The listing builds one solid part. Answer for the finished solid, in the listing's coordinates (mm). Round coordinates to 2 decimals unless told otherwise and drop trailing zeros. Order: outer loops, then holes, each group sorted by start corner. A loop starts at its lowest first (then second) coordinate and runs counter-clockwise, first axis right, second up. Notation, with made-up numbers: (42, 64) - (76, 64) arc R32 cw to (76, 95) - close; hole circle Ø9 at (-12.5, 8.5). An arc over 180 degrees is marked (long way). One line per item, written item: value. Start each with the question number.
1. Flat-ended cylindrical pins translate along their axes: P1, Ø1.7, axis at y = 5, z = -5.5, coming from the +X side; P2, Ø6, axis at y = 6.5, z = 10, coming from the +X side; P3, Ø2.5, axis at y = 7.5, z = -5.5, coming from the -X side. Find the tip coordinate at first contact, or state that the pin passes through.
2. Straight lines are drawn through the part: line 1 (Z direction, x = 0, y = 2.5) (3 decimals); line 2 (X direction, y = 2.75, z = 0) (3 decimals); line 3 (X direction, y = 8, z = -3). For each, find the intervals that lie inside material, in ascending order.
3. For a pull along Z with two mould halves and no side action, classify faces 1 (the flat face through (0, 5, -6.731)), 2 (the flat face through (-8, 7.29, 8)) as released by +Z, released by -Z, zero draft, split by the parting line, or undercut.
4. Section B-B, the plane x = -1 is taken. Give the vertices of the cut face in (y, z).
5. Section A-A, the plane y = 0.5 is taken. Give the vertices of the cut face in (x, z) (3 decimals).
6. Section D-D, the plane x = -10 is taken. Give the vertices of the cut face in (y, z), then the cut area to 3 significant figures.
7. Section C-C, the plane z = 0.5 is taken. Give the vertices of the cut face in (x, y), then the cut area to 3 significant figures.
from build123d import *

# Parameters (mm, degrees)
SKETCH2_R           = 10.795
BOSS_EXTRUDE1_DEPTH = 10.287
SKETCH3_R           = 17.8689
BOSS_EXTRUDE2_DEPTH = 2.9972
CUT_EXTRUDE1_DEPTH  = 11.287
CUT_EXTRUDE2_DEPTH  = 11.287


with BuildPart() as part:
    # Sketch2 → Boss-Extrude1 (new body)
    with BuildSketch(Plane(origin=(0, 0, 0), x_dir=(1, 0, 0), z_dir=(0, 1, 0))):
        Circle(SKETCH2_R)
    extrude(amount=BOSS_EXTRUDE1_DEPTH)

    # Sketch3 → Boss-Extrude2 (add)
    with BuildSketch(Plane(origin=(0, 10.287, 0), x_dir=(1, 0, 0), z_dir=(0, 1, 0))):
        Circle(SKETCH3_R)
    extrude(amount=-BOSS_EXTRUDE2_DEPTH)

    # Sketch4 → Cut-Extrude1 (cut, through all)
    with BuildSketch(Plane(origin=(0, 10.287, 0), x_dir=(1, 0, 0), z_dir=(0, 1, 0))):
        with BuildLine():
            ThreePointArc((1.4e-08, 17.8689), (1.079645228, 17.410056336), (1.4986, 16.314315402))
            ThreePointArc((1.4986, 16.314315402), (3.196164746, 16.068205249), (4.858692347, 15.645951479))
            ThreePointArc((4.858692347, 15.645951479), (5.665077892, 16.497957009), (6.838131777, 16.508711064))
            ThreePointArc((6.838131777, 16.508711064), (3.486049352, 17.525554117), (1.4e-08, 17.8689))
        make_face()
        with BuildLine():
            ThreePointArc((4.858692347, 15.645951479), (3.196164746, 16.068205249), (1.4986, 16.314315402))
            ThreePointArc((1.4986, 16.314315402), (2.893978636, 14.549013087), (4.858692347, 15.645951479))
        make_face()
        with BuildLine():
            ThreePointArc((12.63522035, 12.635220375), (9.927428836, 14.857447422), (6.838131777, 16.508711064))
            ThreePointArc((6.838131777, 16.508711064), (7.660002201, 15.671632478), (7.627744082, 14.498972695))
            ThreePointArc((7.627744082, 14.498972695), (9.101907128, 13.621966658), (10.476292829, 12.595633274))
            ThreePointArc((10.476292829, 12.595633274), (11.547344433, 13.074193358), (12.63522035, 12.635220375))
        make_face()
        with BuildLine():
            ThreePointArc((10.476292829, 12.595633274), (9.101907128, 13.621966658), (7.627744082, 14.498972695))
            ThreePointArc((7.627744082, 14.498972695), (8.241353895, 12.334057732), (10.476292829, 12.595633274))
        make_face()
        with BuildLine():
            ThreePointArc((16.508710924, 6.838132115), (14.857447311, 9.927429003), (12.63522035, 12.635220375))
            ThreePointArc((12.63522035, 12.635220375), (13.074193359, 11.54734445), (12.595633274, 10.476292829))
            ThreePointArc((12.595633274, 10.476292829), (13.621966658, 9.101907128), (14.498972695, 7.627744082))
            ThreePointArc((14.498972695, 7.627744082), (15.671632308, 7.660002268), (16.508710924, 6.838132115))
        make_face()
        with BuildLine():
            ThreePointArc((14.498972695, 7.627744082), (13.621966658, 9.101907128), (12.595633274, 10.476292829))
            ThreePointArc((12.595633274, 10.476292829), (12.334057732, 8.241353895), (14.498972695, 7.627744082))
        make_face()
        with BuildLine():
            ThreePointArc((17.8689, 0), (17.525554083, 3.486049525), (16.508710924, 6.838132115))
            ThreePointArc((16.508710924, 6.838132115), (16.497957082, 5.665078059), (15.645951479, 4.858692347))
            ThreePointArc((15.645951479, 4.858692347), (16.068205249, 3.196164746), (16.314315402, 1.4986))
            ThreePointArc((16.314315402, 1.4986), (17.410056341, 1.079645223), (17.8689, 0))
        make_face()
        with BuildLine():
            ThreePointArc((16.314315402, 1.4986), (16.068205249, 3.196164746), (15.645951479, 4.858692347))
            ThreePointArc((15.645951479, 4.858692347), (14.549013087, 2.893978636), (16.314315402, 1.4986))
        make_face()
        with BuildLine():
            ThreePointArc((16.508710924, -6.838132115), (17.525554083, -3.486049525), (17.8689, 0))
            ThreePointArc((17.8689, 0), (17.410056341, -1.079645223), (16.314315402, -1.4986))
            ThreePointArc((16.314315402, -1.4986), (16.068205249, -3.196164746), (15.645951479, -4.858692347))
            ThreePointArc((15.645951479, -4.858692347), (16.497957082, -5.665078059), (16.508710924, -6.838132115))
        make_face()
        with BuildLine():
            ThreePointArc((15.645951479, -4.858692347), (16.068205249, -3.196164746), (16.314315402, -1.4986))
            ThreePointArc((16.314315402, -1.4986), (14.549013087, -2.893978636), (15.645951479, -4.858692347))
        make_face()
        with BuildLine():
            ThreePointArc((12.635220358, -12.635220367), (14.857447314, -9.927428998), (16.508710924, -6.838132115))
            ThreePointArc((16.508710924, -6.838132115), (15.671632308, -7.660002268), (14.498972695, -7.627744082))
            ThreePointArc((14.498972695, -7.627744082), (13.621966658, -9.101907128), (12.595633274, -10.476292829))
            ThreePointArc((12.595633274, -10.476292829), (13.074193359, -11.547344445), (12.635220358, -12.635220367))
        make_face()
        with BuildLine():
            ThreePointArc((12.595633274, -10.476292829), (13.621966658, -9.101907128), (14.498972695, -7.627744082))
            ThreePointArc((14.498972695, -7.627744082), (12.334057732, -8.241353895), (12.595633274, -10.476292829))
        make_face()
        with BuildLine():
            ThreePointArc((6.838132083, -16.508710938), (9.927428978, -14.857447327), (12.635220358, -12.635220367))
            ThreePointArc((12.635220358, -12.635220367), (11.547344438, -13.074193358), (10.476292829, -12.595633274))
            ThreePointArc((10.476292829, -12.595633274), (9.101907128, -13.621966658), (7.627744082, -14.498972695))
            ThreePointArc((7.627744082, -14.498972695), (7.660002262, -15.671632324), (6.838132083, -16.508710938))
        make_face()
        with BuildLine():
            ThreePointArc((7.627744082, -14.498972695), (9.101907128, -13.621966658), (10.476292829, -12.595633274))
            ThreePointArc((10.476292829, -12.595633274), (8.241353895, -12.334057732), (7.627744082, -14.498972695))
        make_face()
        with BuildLine():
            ThreePointArc((0, -17.8689), (3.486049507, -17.525554087), (6.838132083, -16.508710938))
            ThreePointArc((6.838132083, -16.508710938), (5.665078043, -16.497957075), (4.858692347, -15.645951479))
            ThreePointArc((4.858692347, -15.645951479), (3.196164746, -16.068205249), (1.4986, -16.314315402))
            ThreePointArc((1.4986, -16.314315402), (1.079645223, -17.410056341), (0, -17.8689))
        make_face()
        with BuildLine():
            ThreePointArc((1.4986, -16.314315402), (3.196164746, -16.068205249), (4.858692347, -15.645951479))
            ThreePointArc((4.858692347, -15.645951479), (2.893978636, -14.549013087), (1.4986, -16.314315402))
        make_face()
        with BuildLine():
            ThreePointArc((-4.858692347, -15.645951479), (-5.665078063, -16.497957083), (-6.838132123, -16.508710921))
            ThreePointArc((-6.838132123, -16.508710921), (-3.486049529, -17.525554082), (0, -17.8689))
            ThreePointArc((0, -17.8689), (-1.079645223, -17.410056341), (-1.4986, -16.314315402))
            ThreePointArc((-1.4986, -16.314315402), (-3.196164746, -16.068205249), (-4.858692347, -15.645951479))
        make_face()
        with BuildLine():
            ThreePointArc((-1.4986, -16.314315402), (-2.893978636, -14.549013087), (-4.858692347, -15.645951479))
            ThreePointArc((-4.858692347, -15.645951479), (-3.196164746, -16.068205249), (-1.4986, -16.314315402))
        make_face()
        with BuildLine():
            ThreePointArc((-7.627744082, -14.498972695), (-8.241353895, -12.334057732), (-10.476292829, -12.595633274))
            ThreePointArc((-10.476292829, -12.595633274), (-9.101907128, -13.621966658), (-7.627744082, -14.498972695))
        make_face()
        with BuildLine():
            ThreePointArc((-14.498972695, -7.627744082), (-15.671632446, -7.660002214), (-16.508711038, -6.838131842))
            ThreePointArc((-16.508711038, -6.838131842), (-14.857447398, -9.927428873), (-12.635220362, -12.635220362))
            ThreePointArc((-12.635220362, -12.635220362), (-13.074193358, -11.547344441), (-12.595633274, -10.476292829))
            ThreePointArc((-12.595633274, -10.476292829), (-13.621966658, -9.101907128), (-14.498972695, -7.627744082))
        make_face()
        with BuildLine():
            ThreePointArc((-12.595633274, -10.476292829), (-12.334057732, -8.241353895), (-14.498972695, -7.627744082))
            ThreePointArc((-14.498972695, -7.627744082), (-13.621966658, -9.101907128), (-12.595633274, -10.476292829))
        make_face()
        with BuildLine():
            ThreePointArc((-16.314315402, -1.4986), (-17.410056347, -1.079645218), (-17.8689, 1.4e-08))
            ThreePointArc((-17.8689, 1.4e-08), (-17.525554113, -3.486049372), (-16.508711038, -6.838131842))
            ThreePointArc((-16.508711038, -6.838131842), (-16.497957023, -5.665077924), (-15.645951479, -4.858692347))
            ThreePointArc((-15.645951479, -4.858692347), (-16.068205249, -3.196164746), (-16.314315402, -1.4986))
        make_face()
        with BuildLine():
            ThreePointArc((-15.645951479, -4.858692347), (-14.549013087, -2.893978636), (-16.314315402, -1.4986))
            ThreePointArc((-16.314315402, -1.4986), (-16.068205249, -3.196164746), (-15.645951479, -4.858692347))
        make_face()
        with BuildLine():
            ThreePointArc((-15.645951479, 4.858692347), (-16.497957093, 5.665078085), (-16.508710903, 6.838132168))
            ThreePointArc((-16.508710903, 6.838132168), (-17.525554076, 3.486049559), (-17.8689, 1.4e-08))
            ThreePointArc((-17.8689, 1.4e-08), (-17.410056336, 1.079645228), (-16.314315402, 1.4986))
            ThreePointArc((-16.314315402, 1.4986), (-16.068205249, 3.196164746), (-15.645951479, 4.858692347))
        make_face()
        with BuildLine():
            ThreePointArc((-16.314315402, 1.4986), (-14.549013087, 2.893978636), (-15.645951479, 4.858692347))
            ThreePointArc((-15.645951479, 4.858692347), (-16.068205249, 3.196164746), (-16.314315402, 1.4986))
        make_face()
        with BuildLine():
            ThreePointArc((-12.595633274, 10.476292829), (-13.074193358, 11.547344436), (-12.63522037, 12.635220355))
            ThreePointArc((-12.63522037, 12.635220355), (-14.857447303, 9.927429015), (-16.508710903, 6.838132168))
            ThreePointArc((-16.508710903, 6.838132168), (-15.671632282, 7.660002279), (-14.498972695, 7.627744082))
            ThreePointArc((-14.498972695, 7.627744082), (-13.621966658, 9.101907128), (-12.595633274, 10.476292829))
        make_face()
        with BuildLine():
            ThreePointArc((-14.498972695, 7.627744082), (-12.334057732, 8.241353895), (-12.595633274, 10.476292829))
            ThreePointArc((-12.595633274, 10.476292829), (-13.621966658, 9.101907128), (-14.498972695, 7.627744082))
        make_face()
        with BuildLine():
            ThreePointArc((-7.627744082, 14.498972695), (-7.660002268, 15.671632308), (-6.838132115, 16.508710924))
            ThreePointArc((-6.838132115, 16.508710924), (-9.927429, 14.857447313), (-12.63522037, 12.635220355))
            ThreePointArc((-12.63522037, 12.635220355), (-11.547344447, 13.074193359), (-10.476292829, 12.595633274))
            ThreePointArc((-10.476292829, 12.595633274), (-9.101907128, 13.621966658), (-7.627744082, 14.498972695))
        make_face()
        with BuildLine():
            ThreePointArc((-10.476292829, 12.595633274), (-8.241353895, 12.334057732), (-7.627744082, 14.498972695))
            ThreePointArc((-7.627744082, 14.498972695), (-9.101907128, 13.621966658), (-10.476292829, 12.595633274))
        make_face()
        with BuildLine():
            ThreePointArc((-4.858692347, 15.645951479), (-2.893978636, 14.549013087), (-1.4986, 16.314315402))
            ThreePointArc((-1.4986, 16.314315402), (-3.196164746, 16.068205249), (-4.858692347, 15.645951479))
        make_face()
        with BuildLine():
            ThreePointArc((-1.4986, 16.314315402), (-1.079645218, 17.410056347), (1.4e-08, 17.8689))
            ThreePointArc((1.4e-08, 17.8689), (-3.486049518, 17.525554085), (-6.838132115, 16.508710924))
            ThreePointArc((-6.838132115, 16.508710924), (-5.665078059, 16.497957082), (-4.858692347, 15.645951479))
            ThreePointArc((-4.858692347, 15.645951479), (-3.196164746, 16.068205249), (-1.4986, 16.314315402))
        make_face()
        with BuildLine():
            ThreePointArc((-10.476292829, -12.595633274), (-11.547344441, -13.074193358), (-12.635220362, -12.635220362))
            ThreePointArc((-12.635220362, -12.635220362), (-9.927428999, -14.857447314), (-6.838132123, -16.508710921))
            ThreePointArc((-6.838132123, -16.508710921), (-7.66000227, -15.671632304), (-7.627744082, -14.498972695))
            ThreePointArc((-7.627744082, -14.498972695), (-9.101907128, -13.621966658), (-10.476292829, -12.595633274))
        make_face()
    extrude(amount=-CUT_EXTRUDE1_DEPTH, mode=Mode.SUBTRACT)

    # Sketch5 → Cut-Extrude2 (cut, through all)
    with BuildSketch(Plane(origin=(0, 10.287, 0), x_dir=(1, 0, 0), z_dir=(0, 1, 0))):
        with BuildLine():
            Line((-1.9431, 4.597329834), (-1.9431, 6.731))
            Line((-1.9431, 6.731), (1.9431, 6.731))
            Line((1.9431, 6.731), (1.9431, 4.597329834))
            ThreePointArc((1.9431, 4.597329834), (0, -4.9911), (-1.9431, 4.597329834))
        make_face()
    extrude(amount=-CUT_EXTRUDE2_DEPTH, mode=Mode.SUBTRACT)


solid = part.part
Answer list:
1. P1: stops at x = 9.74
1. P2: stops at x = 16.36
1. P3: stops at x = -16.62
2. line 1: z = -10.795 to -6.731, 4.991 to 10.795
2. line 2: x = -10.795 to -4.991, 4.991 to 10.795
2. line 3: x = -14.53 to -3.99, 3.99 to 14.53
3. face 1: undercut
3. face 2: zero draft
4. outline: (0, -10.75) - (7.29, -10.75) - (7.29, -17.49) - (10.29, -17.49) - (10.29, -6.73) - (0, -6.73) - close; (0, 4.89) - (10.29, 4.89) - (10.29, 17.49) - (7.29, 17.49) - (7.29, 10.75) - (0, 10.75) - close
5. outline: circle Ø21.59 at (0, 0); hole (-1.943, -6.731) - (1.943, -6.731) - (1.943, -4.597) arc R4.991 ccw (long way) to (-1.943, -4.597) - close
6. outline: (0, -4.07) - (7.29, -4.07) - (7.29, -12.23) - (10.29, -12.23) - (10.29, 12.23) - (7.29, 12.23) - (7.29, 4.07) - (0, 4.07) - close
6. area: 133 mm²
7. outline: (-17.78, 7.29) - (-10.78, 7.29) - (-10.78, 0) - (-4.97, 0) - (-4.97, 10.29) - (-17.78, 10.29) - close; (4.97, 0) - (10.78, 0) - (10.78, 7.29) - (17.78, 7.29) - (17.78, 10.29) - (4.97, 10.29) - close
7. area: 162 mm²
